Design review of the part built by this model. Coordinates are the model's own, in mm. Face numbers are marked on the shaded views. A direction names the side the tool comes from. Give positions to 0.01 mm unless a question says otherwise; leave off trailing zeros. Loops run counter-clockwise (first coordinate to the right, second up) from the corner with the lowest first, then second, coordinate; pieces in that order, holes last. Notation, with made-up numbers: M 64.25,54 L 121.25,54 A19 cw 121.25,82 Z; hole C -34,57 d7. An arc over 180 degrees is marked long. Use a Markdown table: item, result. Add a question column.
(1) Add section D-D, the plane y = 5.5. Give the boundary of the cut face in (x, z) (3 decimals).
(2) Draft analysis for pull direction Z (two halves, no side actions). For the marked faces 5, 6, 7 and 8, state which applies: pulls with the +Z half, pulls with the -Z half, needs draft (parallel to the pull), parting line crosses it, or undercut.
(3) For the marked faces 1, 2, 3 and 4, list the 3-axis set-ups (+Z, -Z, +X, -X, +Y, -Y) from which the entire face can be reached by the end or side of a thin tool; tool diameter is ignored.
(4) Insertion check: pin 1 Ø1.5 at (y, z) = (3, -2.5) entering from +X; pin 2 Ø1.5 at (x, y) = (5, 6) entering from -Z (3 decimals); pin 3 Ø1.9 at (y, z) = (2.5, -5) entering from -X; pin 4 Ø2.5 at (y, z) = (1.5, -6) entering from -X. Each pin has a flat end and moves straight along its axis. Give the tip position at first contact, or say it passes through.
(5) Add section A-A, the plane y = 2. Give the boundary of the cut face in (x, z) (3 decimals), then the cut area to 3 significant figures.
(6) Add section B-B, the plane x = 2. Give the boundary of the cut face in (y, z) (3 decimals).
(7) Add section C-C, the plane z = -6.75. Give the boundary of the cut face in (x, y), then the cut area to 3 significant figures.
(8) For probe 1 along Z at (x, y) = (2.5, 0.5) (3 decimals); probe 2 along X at (y, z) = (4.25, -5); probe 3 along Z at (x, y) = (5.25, 6.5), list the stretches that pass through material, from the lowest coordinate up.
```python
from build123d import *

# Parameters (mm, degrees)
SKICA1_W                 = 7
SKICA1_H                 = 12
SKICA1_W_2               = 2.46
SKICA1_H_2               = 2.37
P_IDAT_VYSUNUT_M1_DEPTH  = 0.46
SKICA2_W                 = 4.88
SKICA2_H                 = 6.39
SKICA2_W_2               = 2.46
SKICA2_H_2               = 2.37
P_IDAT_VYSUNUT_M2_DEPTH  = 4
SKICA3_W                 = 4.88
SKICA3_H                 = 6.39
P_IDAT_VYSUNUT_M3_DEPTH  = 2.8
ODEBRAT_VYSUNUT_M1_DEPTH = 10


with BuildPart() as part:
    # Skica1 → Přidat vysunutím1 (new body)
    with BuildSketch(Plane(origin=(0, 0, 0), x_dir=(1, 0, 0), z_dir=(0, 1, 0))):
        with Locations((3.5, 6)):
            Rectangle(SKICA1_W, SKICA1_H)
        with Locations((3.5, 6)):
            Rectangle(SKICA1_W_2, SKICA1_H_2, mode=Mode.SUBTRACT)
    extrude(amount=P_IDAT_VYSUNUT_M1_DEPTH)

    # Skica2 → Přidat vysunutím2 (add)
    with BuildSketch(Plane(origin=(0, 0.46, 0), x_dir=(1, 0, 0), z_dir=(0, 1, 0))):
        with Locations((3.5, 6)):
            Rectangle(SKICA2_W, SKICA2_H)
        with Locations((3.5, 6)):
            Rectangle(SKICA2_W_2, SKICA2_H_2, mode=Mode.SUBTRACT)
    extrude(amount=P_IDAT_VYSUNUT_M2_DEPTH)

    # Skica3 → Přidat vysunutím3 (add)
    with BuildSketch(Plane(origin=(0, 4.46, 0), x_dir=(1, 0, 0), z_dir=(0, 1, 0))):
        with Locations((3.5, 6)):
            Rectangle(SKICA3_W, SKICA3_H)
    extrude(amount=P_IDAT_VYSUNUT_M3_DEPTH)

    # Skica4 → Odebrat vysunutím1 (cut)
    with BuildSketch(Plane.ZY.offset(-1.06)):
        Polygon((-9.195, 7.26), (-9.195, 6.26), (-8.024764385, 7.26), align=None)
        Polygon((-6, 7.26), (-8.024764385, 7.26), (-7.170235615, 6.26), align=None)
        Polygon((-3.975235615, 7.26), (-6, 7.26), (-5.145471231, 6.26), align=None)
        Polygon((-2.805, 7.26), (-3.975235615, 7.26), (-2.805, 6.26), align=None)
    extrude(amount=-ODEBRAT_VYSUNUT_M1_DEPTH, mode=Mode.SUBTRACT)


solid = part.part
```
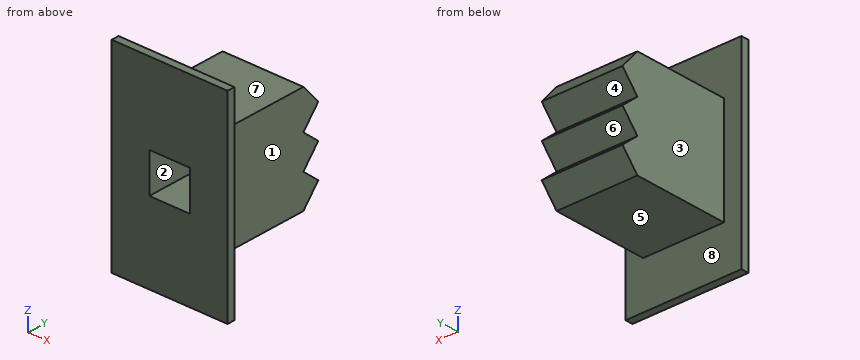
Established:
| question | item | result |
|---|---|---|
| 1 | outline | M 1.06,-9.195 L 5.94,-9.195 L 5.94,-2.805 L 1.06,-2.805 Z |
| 2 | face 5 | pulls with the -Z half |
| 2 | face 6 | undercut |
| 2 | face 7 | pulls with the +Z half |
| 2 | face 8 | needs draft |
| 3 | face 1 | +Z, -Z, +X, +Y |
| 3 | face 2 | -Y |
| 3 | face 3 | +Z, -Z, -X, +Y |
| 3 | face 4 | +X, -X, +Y |
| 4 | pin 1 | x = 5.94 |
| 4 | pin 2 | z = -9.195 |
| 4 | pin 3 | x = 1.06 |
| 4 | pin 4 | x = 0 |
| 5 | outline | M 1.06,-9.195 L 5.94,-9.195 L 5.94,-2.805 L 1.06,-2.805 Z; hole M 2.27,-7.185 L 4.73,-7.185 L 4.73,-4.815 L 2.27,-4.815 Z |
| 5 | area | 25.4 mm^2 |
| 6 | outline | M 0,-12 L 0.46,-12 L 0.46,-9.195 L 6.26,-9.195 L 7.26,-8.025 L 6.26,-7.17 L 7.26,-6 L 6.26,-5.145 L 7.26,-3.975 L 6.26,-2.805 L 0.46,-2.805 L 0.46,0 L 0,0 Z |
| 7 | outline | M 0,0 L 2.27,0 L 2.27,4.46 L 4.73,4.46 L 4.73,0 L 7,0 L 7,0.46 L 5.94,0.46 L 5.94,6.62 L 1.06,6.62 L 1.06,0.46 L 0,0.46 Z |
| 7 | area | 22.3 mm^2 |
| 8 | probe 1 | -9.195 to -7.185, -4.815 to -2.805 |
| 8 | probe 2 | 1.06 to 2.27, 4.73 to 5.94 |
| 8 | probe 3 | -8.91 to -7.38, -6.89 to -5.35, -4.86 to -3.09 |
